Source: CAD feature listing. Evaluate the final solid. Frame: model axes, mm. Face numbers are marked on the shaded views. A direction names the side the tool comes from. Give positions to 0.01 mm unless a question says otherwise; leave off trailing zeros. Order: outer loops, then holes, each group sorted by start corner. A loop starts at its lowest first (then second) coordinate and runs counter-clockwise, first axis right, second up. Notation, with made-up numbers: (23.25, 42.25) -> (38.25, 42.25) arc R9 cw to (38.25, 47.25) -> close; hole circle Ø1 at (-33.5, -28.75). An arc over 180 degrees is marked (long way). Answer in a Markdown table with one row per item.
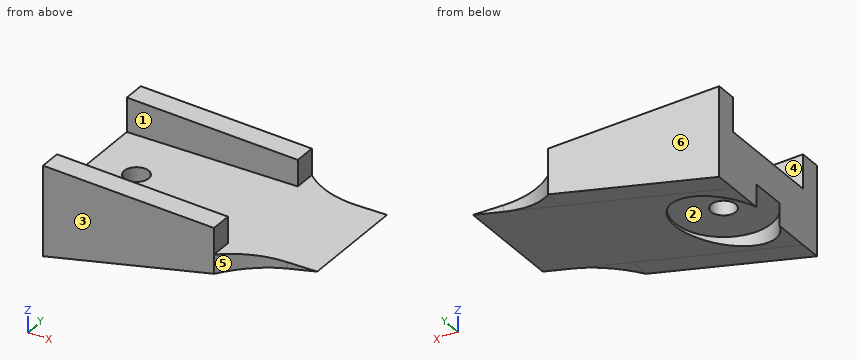
```python
from build123d import *

# Parameters (mm, degrees)
EXTRUDE_1_DEPTH     = 15
SKETCH_3_R          = 6.5
CUT_EXTRUDE_2_DEPTH = 3
SKETCH_4_R          = 1.65
CUT_EXTRUDE_3_DEPTH = 39.336783637
EXTRUDE_2_DEPTH     = 3
FILLET_1_R          = 12


with BuildPart() as part:
    # 草图2 → 凸台-拉伸1 (new body)
    with BuildSketch(Plane(origin=(0, 0, 0), x_dir=(1, 0, 0), z_dir=(0, 1, 0))):
        Polygon((0, 0), (35, 0), (0, 7.439479658), align=None)
    extrude(amount=EXTRUDE_1_DEPTH)

    # 草图3 → 切除-拉伸2 (cut)
    with BuildSketch(Plane.XY.offset(-7.439479658)):
        with Locations((6, 7.5)):
            Circle(SKETCH_3_R)
    extrude(amount=CUT_EXTRUDE_2_DEPTH, mode=Mode.SUBTRACT)

    # 草图4 → 切除-拉伸3 (cut, through all)
    with BuildSketch(Plane(origin=(0, 0, -4.439479658), x_dir=(-1, 0, 0), z_dir=(0, 0, -1))):
        with Locations((-6, 7.5)):
            Circle(SKETCH_4_R)
    extrude(amount=-CUT_EXTRUDE_3_DEPTH, mode=Mode.SUBTRACT)

    # 草图6 → 凸台-拉伸2 (add)
    with BuildSketch(Plane(origin=(0, 15, 0), x_dir=(1, 0, 0), z_dir=(0, 1, 0))):
        Polygon((0, 7.439479658), (0, -4.560520342), (23, -3.520495202), (23, 2.55067874), align=None)
    extrude_2 = extrude(amount=EXTRUDE_2_DEPTH)

    # 镜向1: 凸台-拉伸2 across plane
    add(extrude_2.mirror(Plane(origin=(0, 7.5, 0), x_dir=(0, 0, 1), z_dir=(0, -1, 0))))

    # 圆角1
    # the kernel refuses this fillet: 12 mm, written as the material it adds along each edge
    with BuildSketch(Plane(origin=(23, 0, 0), x_dir=(0, -1, 0), z_dir=(0, 0, -1))) as fillet_1_piece_1_section:
        with BuildLine():
            CenterArc((12, -7.937253933), FILLET_1_R, 138.590377891, 41.409622109)
            Line((0, -7.937253933), (0, 0))
            Line((0, 0), (3, 0))
        make_face()
    fillet_1_piece_1 = extrude(amount=22.393813573, mode=Mode.PRIVATE)
    fillet_1_piece_1 = split(fillet_1_piece_1, bisect_by=Plane(origin=(26.786150339, -0.752577895, -1.745907642), z_dir=(-0.20791169081775981, 0, 0.9781476007338056)), keep=Keep.TOP, mode=Mode.PRIVATE)
    add(fillet_1_piece_1)
    with BuildSketch(Plane(origin=(23, 15, 0), x_dir=(0, 1, 0), z_dir=(0, 0, -1))) as fillet_1_piece_2_section:
        with BuildLine():
            CenterArc((12, 7.937253933), FILLET_1_R, 180, 41.409622109)
            Line((0, 7.937253933), (0, 0))
            Line((0, 0), (3, 0))
        make_face()
    fillet_1_piece_2 = extrude(amount=22.393813573, mode=Mode.PRIVATE)
    fillet_1_piece_2 = split(fillet_1_piece_2, bisect_by=Plane(origin=(26.786150339, 15.752577895, -1.745907642), z_dir=(-0.20791169081775981, 0, 0.9781476007338056)), keep=Keep.TOP, mode=Mode.PRIVATE)
    add(fillet_1_piece_2)


solid = part.part
```
(1) Pull-direction query (Y, two-part tool) for the marked faces 4, 5 and 6; classes: +Y half, -Y half, draft (parallel to the pull), parting line (faces both ways), or undercut.
A:
| item | result |
|---|---|
| face 4 | undercut |
| face 5 | -Y half |
| face 6 | +Y half |
(2) First-contact query: pin 1 Ø5.5 at (x, y) = (6, 7.5) entering from -Z; pin 2 Ø5 at (x, y) = (16.5, 5) entering from -Z; pin 3 Ø1 at (x, y) = (6, 5) entering from +Z. Flat tips, straight axial feed; report the tip coordinate or a pass-through.
A:
| item | result |
|---|---|
| pin 1 | stops at z = -4.44 |
| pin 2 | stops at z = -4.46 |
| pin 3 | stops at z = 0 |
(3) Ray query, probe 1 along Y at (x, z) = (6.5, 1.75); probe 2 along Y at (x, z) = (6, -5.4); probe 3 along Z at (x, y) = (10.5, 8). Return the intervals inside material, ascending.
A:
| item | result |
|---|---|
| probe 1 | y = -3 to 0, 15 to 18 |
| probe 2 | y = -3 to 1, 14 to 18 |
| probe 3 | z = -4.44 to 0 |
(4) Section query B-B (x = 6). Return the cut outline in (y, z), plus the area to 3 significant figures.
A:
| item | result |
|---|---|
| outline | (-3, -6.16) -> (1, -6.16) -> (1, -4.44) -> (5.85, -4.44) -> (5.85, 0) -> (0, 0) -> (0, 4.29) -> (-3, 4.29) -> close; (9.15, -4.44) -> (14, -4.44) -> (14, -6.16) -> (18, -6.16) -> (18, 4.29) -> (15, 4.29) -> (15, 0) -> (9.15, 0) -> close |
| area | 118 mm^2 |
(5) Section query A-A (y = 7.5). Return the cut outline in (x, z), plus the area to 3 significant figures.
A:
| item | result |
|---|---|
| outline | (0, -4.44) -> (4.35, -4.44) -> (4.35, 0) -> (0, 0) -> close; (7.65, -4.44) -> (12.5, -4.44) -> (12.5, -4.78) -> (35, 0) -> (7.65, 0) -> close |
| area | 94.6 mm^2 |
(6) Section query D-D (x = 10.5). Return the cut outline in (y, z), plus the area to 3 significant figures.
A:
| item | result |
|---|---|
| outline | (-3, -5.21) -> (2.81, -5.21) -> (2.81, -4.44) -> (12.19, -4.44) -> (12.19, -5.21) -> (18, -5.21) -> (18, 4.09) -> (15, 4.09) -> (15, 0) -> (0, 0) -> (0, 4.09) -> (-3, 4.09) -> close |
| area | 127 mm^2 |
(7) Section query C-C (z = -6.5). Return the cut outline in (x, y), plus the area to 3 significant figures.
A:
| item | result |
|---|---|
| outline | (0, -3) -> (4.42, -3) -> (4.42, 1.19) arc R6.5 cw to (0, 5) -> close; (0, 10) arc R6.5 cw to (4.42, 13.81) -> (4.42, 18) -> (0, 18) -> close |
| area | 48.5 mm^2 |
(8) Access query for the marked faces 1, 2 and 3. Directions: +Z, -Z, +X, -X, +Y, -Y. A direction counts if a zero-diameter tool reaches every point of the face in a straight line with its end or side. Return the directions, or none.
A:
| item | result |
|---|---|
| face 1 | +Z, +X, -X |
| face 2 | -Z |
| face 3 | +Z, -Z, +X, -X, -Y |
